Can you work these out from the model? Positions are in its coordinate system, mm. A direction names the side the tool comes from. Give positions to 0.01 mm unless a question says otherwise; leave off trailing zeros. Write each loop counter-clockwise with the first axis right and the second up, starting at its lowest first coordinate (ties: lowest second). Pieces come first, ordered by that corner, then holes. Notation, with made-up numbers: M 19.25,59 L 43.25,59 A24 ccw 43.25,83 Z; hole C 45,-26.75 d10. An arc over 180 degrees is marked long. Write each question's results on one line, items separated by ' | '.
from build123d import *

# Parameters (mm, degrees)
SCHNITT_LINEAR_AUSTRAGEN1_REACH = 11
SKIZZE2_W                       = 6.040100504
SKIZZE2_H                       = 0.8


with BuildPart() as part:
    # Skizze1 → Rotation1 (revolve)
    with BuildSketch(Plane.XY):
        Polygon((0, 4), (9, 4), (9, 5), (1.535898385, 7), (0, 7), align=None)
    revolve(axis=Axis((0, 0, 0), (1, 0, 0)))

    # Skizze2 → Schnitt-Linear austragen1 (cut, up to next)
    with BuildSketch(Plane(origin=(0, 0, 0), x_dir=(0, 0, -1), z_dir=(1, 0, 0)), mode=Mode.PRIVATE) as schnitt_linear_austragen1_sk1:
        with Locations((-7, 0)):
            Rectangle(SKIZZE2_W, SKIZZE2_H)
    schnitt_linear_austragen1_tool1 = extrude(schnitt_linear_austragen1_sk1.sketch, amount=SCHNITT_LINEAR_AUSTRAGEN1_REACH, mode=Mode.PRIVATE) & part.part
    add(schnitt_linear_austragen1_tool1.solids().sort_by_distance((0, 0, 7))[0], mode=Mode.SUBTRACT)


solid = part.part
Item 1: I want a section at A-A, the plane y = 0. Please give me the cut outline in (x, z).
Geometry says:
outline: M 0,-7 L 1.54,-7 L 9,-5 L 9,-4 L 0,-4 Z
Item 2: I want a section at C-C, the plane x = 4.25. Please give me the cut outline in (y, z), and give its area (3 significant figures).
Geometry says:
outline: M -0.4,3.98 L -0.4,6.26 A6.27 ccw long 0.4,6.26 L 0.4,3.98 A4 cw long Z | area: 71.5 mm2
Item 3: Thinking about a two-plate mould opening in Y: for faces 3 (the face through (9, 2, 4)), 4 (the face through (3, -0.4, 5)), which applies, +Y half, -Y half, draft (parallel to the pull), parting line (faces both ways), or undercut?
Geometry says:
face 3: draft | face 4: undercut
Item 4: I'm going to push flat-ended pins straight in: pin 1 (5 mm diameter, centred on y = 0, z = 0, fed in from -X); pin 2 (2.5 mm diameter, centred on x = 5, z = 6, fed in from +Y); pin 3 (3 mm diameter, centred on x = 6, y = 1.5, fed in from +Z); pin 4 (5 mm diameter, centred on x = 8, z = 0, fed in from +Y). Where does each tip first touch, or does it pass through?
Geometry says:
pin 1: passes through | pin 2: stops at y = 3.87 | pin 3: stops at z = 6.11 | pin 4: stops at y = 5.94
Item 5: I want a section at B-B, the plane x = 1. Please give me the cut outline in (y, z), and give its area (3 significant figures).
Geometry says:
outline: M -0.4,3.98 L -0.4,6.99 A7 ccw long 0.4,6.99 L 0.4,3.98 A4 cw long Z | area: 101 mm2
Item 6: For faces 1 (the face through (3, 0.4, 5)), 2 (the face through (5, 0, -4)), which set-ups out of +Z, -Z, +X, -X, +Y, -Y let a thin tool reach every point of the face, with its end or its side?
Geometry says:
face 1: +Z, +X, -X | face 2: +X, -X
Item 7: If I drill on line 1 (Z direction, x = 8.25, y = 0.75); line 2 (Y direction, x = 4.5, z = 0); line 3 (Z direction, x = 6.5, y = -1), over which ranges is the centre line in solid material (lowest first)? Write a range as from..to.
Geometry says:
line 1: z = -5.15..-3.93, 3.93..5.15 | line 2: y = -6.21..-4, 4..6.21 | line 3: z = -5.58..-3.87, 3.87..5.58
